```python
from build123d import *

# Parameters (mm, degrees)
SKETCH1_W                  = 38.1
SKETCH1_H                  = 38.1
SKETCH1_W_2                = 31.75
SKETCH1_H_2                = 31.75
EXTRUDE1_DEPTH             = 101.6
FILLET1_R                  = 3.175
F_1_2_0_5_DIAMETER_HOLE1_D = 12.7


with BuildPart() as part:
    # Sketch1 → Extrude1 (new body)
    with BuildSketch(Plane.XY):
        Rectangle(SKETCH1_W, SKETCH1_H)
        Rectangle(SKETCH1_W_2, SKETCH1_H_2, mode=Mode.SUBTRACT)
    extrude(amount=EXTRUDE1_DEPTH)

    # Fillet1
    fillet1_edges = [part.edges().sort_by_distance(p)[0] for p in [
        (19.05, -19.05, 50.8),
        (-19.05, -19.05, 50.8),
        (-19.05, 19.05, 50.8),
        (19.05, 19.05, 50.8),
    ]]
    fillet(fillet1_edges, radius=FILLET1_R)

    # 1/2 (0.5) Diameter Hole1 (through all)
    with Locations(Plane.XZ.offset(19.05)):
        with Locations((0, 69.85)):
            Hole(F_1_2_0_5_DIAMETER_HOLE1_D / 2)


solid = part.part
```
Check sheet for the modelled part. Datum: model origin and axes. Units: mm. A direction names the side the tool comes from. Round coordinates to 2 decimals unless told otherwise and drop trailing zeros. Order: outer loops, then holes, each group sorted by start corner. A loop starts at its lowest first (then second) coordinate and runs counter-clockwise, first axis right, second up.
1) Section check D-D (x = 0). Record the boundary of the cut face in (y, z) (3 decimals).
2) Go/stop test with a flat-tipped pin: pin 1 Ø4 at (x, y) = (14.5, -2) entering from +Z. Record where the tip stops, or that it passes through.
3) Mould release check, pull along X, two halves, no side actions. Record for faces 3 (the flat face through (0, -15.875, 50)), 4 (the flat face through (15.875, 0, 50)), 5 (the cylindrical face through (-18.14, -18.1, 51.51)), 6 (the flat face through (0, -19.05, 50)): +X half, -X half, draft (parallel to the pull), parting line (faces both ways), or undercut.
4) Tool access check on faces 1 (the cylindrical face through (18.1, -18.14, 51.51)), 2 (the flat face through (0, 15.875, 50)). Record the directions out of +Z, -Z, +X, -X, +Y, -Y that give a thin tool (end or side, any length) a straight path to the whole face; none if there is none.
5) Section check A-A (x = 8.5). Record the boundary of the cut face in (y, z) (3 decimals), and give its area (3 significant figures).
6) Scan line: line 1 (Y direction, x = -5.5, z = 80.5) (3 decimals). Record every from-to range of solid material in increasing order.
7) Section check B-B (z = 16.5). Record the boundary of the cut face in (x, y) (3 decimals), and give its area (3 significant figures).
Result:
1. outline: (-19.05, 0) - (-15.875, 0) - (-15.875, 63.5) - (-19.05, 63.5) - close; (-19.05, 76.2) - (-15.875, 76.2) - (-15.875, 101.6) - (-19.05, 101.6) - close; (15.875, 0) - (19.05, 0) - (19.05, 63.5) - (15.875, 63.5) - close; (15.875, 76.2) - (19.05, 76.2) - (19.05, 101.6) - (15.875, 101.6) - close
2. pin 1: stops at z = 101.6
3. face 3: undercut
3. face 4: undercut
3. face 5: -X half
3. face 6: draft
4. face 1: +Z, -Z, +X, -Y
4. face 2: +Z, -Z
5. outline: (-19.05, 0) - (-15.875, 0) - (-15.875, 101.6) - (-19.05, 101.6) - close; (15.875, 0) - (19.05, 0) - (19.05, 101.6) - (15.875, 101.6) - close
5. area: 645 mm2
6. line 1: y = -19.05 to -15.875, 15.875 to 19.05
7. outline: (-19.05, -15.875) arc R3.175 ccw to (-15.875, -19.05) - (15.875, -19.05) arc R3.175 ccw to (19.05, -15.875) - (19.05, 15.875) arc R3.175 ccw to (15.875, 19.05) - (-15.875, 19.05) arc R3.175 ccw to (-19.05, 15.875) - close; hole (-15.875, -15.875) - (15.875, -15.875) - (15.875, 15.875) - (-15.875, 15.875) - close
7. area: 435 mm2
